```python
from build123d import *

# Parameters (mm, degrees)
SKETCH1_W           = 85
SKETCH1_H           = 65
BOSS_EXTRUDE1_DEPTH = 1.6
CUT_EXTRUDE1_DEPTH  = 10
SKETCH4_R           = 1.5
CUT_EXTRUDE2_DEPTH  = 16


with BuildPart() as part:
    # Sketch1 → Boss-Extrude1 (new body)
    with BuildSketch(Plane(origin=(0, 0, 0), x_dir=(1, 0, 0), z_dir=(0, 1, 0))):
        Rectangle(SKETCH1_W, SKETCH1_H)
    extrude(amount=BOSS_EXTRUDE1_DEPTH)

    # Sketch3 → Cut-Extrude1 (cut)
    with BuildSketch(Plane(origin=(0, 0, 0), x_dir=(-1, 0, 0), z_dir=(0, -1, 0))):
        Polygon((42.5, 32.5), (42.5, 17.5), (27.5, 32.5), align=None)
        Polygon((27.5, -32.5), (42.5, -32.5), (42.5, -17.5), align=None)
    extrude(amount=-CUT_EXTRUDE1_DEPTH, mode=Mode.SUBTRACT)

    # Sketch4 → Cut-Extrude2 (cut)
    with BuildSketch(Plane(origin=(0, 0, 0), x_dir=(-1, 0, 0), z_dir=(0, -1, 0))):
        with Locations(Location((16.5, -12, 0), (0, 0, 90))):
            Circle(SKETCH4_R)
        with Locations(Location((16.5, 12, 0), (0, 0, 90))):
            Circle(SKETCH4_R)
        with Locations(Location((-39.5, -12, 0), (0, 0, 90))):
            Circle(SKETCH4_R)
        with Locations(Location((-39.5, 12, 0), (0, 0, 90))):
            Circle(SKETCH4_R)
    extrude(amount=-CUT_EXTRUDE2_DEPTH, mode=Mode.SUBTRACT)


solid = part.part
```
Work out the finished part from the listing and answer in its coordinate system (mm). Give positions to 0.01 mm unless a question says otherwise; leave off trailing zeros. Loops run counter-clockwise (first coordinate to the right, second up) from the corner with the lowest first, then second, coordinate; pieces in that order, holes last. Notation, with made-up numbers: (2.5, -32.75) -> (49.5, -32.75) arc R17 cw to (49.5, -5.75) -> close; hole circle Ø11 at (-8, -24). An arc over 180 degrees is marked (long way). One line per question, with ' | ' between items. Start each with the question number.
1) Section B-B, the plane y = 1.1 is taken. Determine the outline of the cut face in (x, z), then the cut area to 3 significant figures.
2) This flat-tipped pin is pushed along its axis until it touches: pin 1 (2.5 mm diameter, centred on x = 39.5, z = -12, fed in from -Y). Where does it stop, or does it pass through?
3) Straight lines are drawn through the part: L1, parallel to X at y = 1.35, z = 12; L2, parallel to Z at x = -31, y = 0.8; L3, parallel to X at y = 0.1, z = -24. For each, find the intervals that lie inside material, in ascending order.
4) Determine the mould class of faces 1 (the face through (-1, 1.6, 0)), 2 (the face through (-16.43, 0.79, 13.5)), 3 (the face through (-35, 1, 25)) for opening direction X: +X half, -X half, draft (parallel to the pull), parting line (faces both ways), or undercut.
5) Section A-A, the plane x = -16.5 is taken. Determine the outline of the cut face in (y, z), then the cut area to 3 significant figures.
6) Section D-D, the plane z = -20 is taken. Determine the outline of the cut face in (x, y), then the cut area to 3 significant figures.
7) Section C-C, the plane z = -12 is taken. Determine the outline of the cut face in (x, y), then the cut area to 3 significant figures.
Resolved:
1) outline: (-42.5, -17.5) -> (-27.5, -32.5) -> (42.5, -32.5) -> (42.5, 32.5) -> (-27.5, 32.5) -> (-42.5, 17.5) -> close; hole circle Ø3 at (-16.5, -12); hole circle Ø3 at (-16.5, 12); hole circle Ø3 at (39.5, -12); hole circle Ø3 at (39.5, 12) | area: 5,270 mm2
2) pin 1: through
3) L1: -42.5 to -18, -15 to 38, 41 to 42.5 | L2: -29 to 29 | L3: -36 to 42.5
4) face 1: draft | face 2: undercut | face 3: -X half
5) outline: (0, -32.5) -> (1.6, -32.5) -> (1.6, -13.5) -> (0, -13.5) -> close; (0, -10.5) -> (1.6, -10.5) -> (1.6, 10.5) -> (0, 10.5) -> close; (0, 13.5) -> (1.6, 13.5) -> (1.6, 32.5) -> (0, 32.5) -> close | area: 94.4 mm2
6) outline: (-40, 0) -> (42.5, 0) -> (42.5, 1.6) -> (-40, 1.6) -> close | area: 132 mm2
7) outline: (-42.5, 0) -> (-18, 0) -> (-18, 1.6) -> (-42.5, 1.6) -> close; (-15, 0) -> (38, 0) -> (38, 1.6) -> (-15, 1.6) -> close; (41, 0) -> (42.5, 0) -> (42.5, 1.6) -> (41, 1.6) -> close | area: 126 mm2
